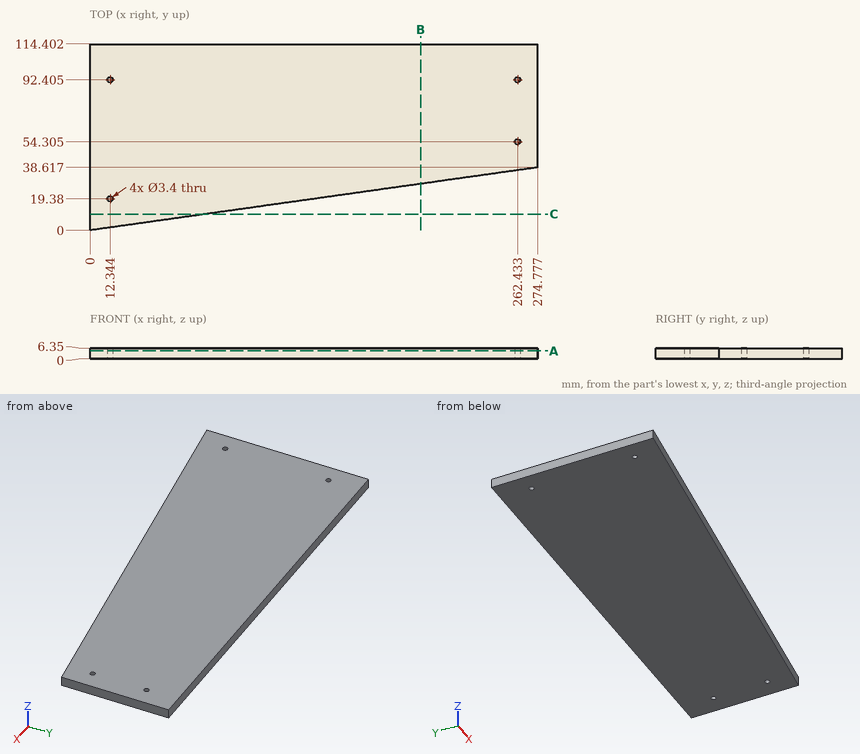
Study the drawing (mm; zero at the part's minimum x, y, z) and answer. Give positions to 0.01 mm unless a question says otherwise; leave off trailing zeros. Write each loop counter-clockwise with the first axis right and the second up, starting at its lowest first coordinate (ties: lowest second). Pieces come first, ordered by that corner, then holes.
(1) The part is cut by section B-B on x = 203. Write down the section's boundary in (y, z), plus the area to 3 significant figures.
Final values:
outline: (28.53, 0) - (114.4, 0) - (114.4, 6.35) - (28.53, 6.35) - close
area: 545 mm2
(2) A flat-ended cylindrical pin translates along its axis: pin 1 Ø1 at (x, z) = (175.5, 1) entering from -Y (1 decimal). Find the tip coordinate at first contact, or state that the pin passes through.
Final values:
pin 1: stops at y = 24.6
(3) The part is cut by section C-C on y = 10. Write down the section's boundary in (x, z).
Final values:
outline: (0, 0) - (71.15, 0) - (71.15, 6.35) - (0, 6.35) - close
(4) The part is cut by section A-A on z = 4.75. Write down the section's boundary in (x, y) (1 decimal), plus the area to 3 significant figures.
Final values:
outline: (0, 0) - (274.8, 38.6) - (274.8, 114.4) - (0, 114.4) - close; hole circle Ø3.4 at (12.3, 19.4); hole circle Ø3.4 at (12.3, 92.4); hole circle Ø3.4 at (262.4, 54.3); hole circle Ø3.4 at (262.4, 92.4)
area: 26,100 mm2
(5) Straight lines are drawn through the part: line 1 (Y direction, x = 262, z = 2); line 2 (Y direction, x = 110.5, z = 0.5); line 3 (Y direction, x = 185.5, z = 4.5). For each, find the intervals that lie inside material, in ascending order.
Final values:
line 1: y = 36.82 to 52.66, 55.95 to 90.76, 94.05 to 114.4
line 2: y = 15.53 to 114.4
line 3: y = 26.07 to 114.4
